Part model, mm, in its own coordinate system. A direction names the side the tool comes from. Round coordinates to 2 decimals unless told otherwise and drop trailing zeros. Write each loop counter-clockwise with the first axis right and the second up, starting at its lowest first coordinate (ties: lowest second). Pieces come first, ordered by that corner, then holes. Notation, with made-up numbers: M 78.25,88.5 L 120.25,88.5 A24 ccw 120.25,101.5 Z; hole C 2,22 d1. An arc over 180 degrees is marked long. Answer as a JSON object with one key per item and string values. Group by question number.
1. Which spindle directions (+Z, -Z, +X, -X, +Y, -Y) get a long thin tool onto all of the face, cutting with end or side? Do faces 4 (the face through (-31.858, -1, 1)), 5 (the face through (9, -21.627, 1)), 6 (the face through (49, 0, 0)). Say none if no direction does.
2. Two-plate mould, pull along X, no slides. Class faces 1 (the face through (-35.154, -0.75, -1.014)), 2 (the face through (47.942, -1, 1)), 3 (the face through (9, 0, -2)): +X half, -X half, draft (parallel to the pull), parting line (faces both ways), or undercut.
3. Band-saw the part on B-B, the plane z = 2. Write the cut outline in (x, y), plus the area to 3 significant figures.
4. Drill centre line: line 1 (X direction, y = -19, z = 1.3). Where is it in solid material? Low to high. Write a range as from..to.
5. Drop flat-ended pins along their axis: pin 1 (1.5 mm diameter, centred on y = -8, z = 1.5, fed in from -X); pin 2 (2.5 mm diameter, centred on x = 51, y = -9, fed in from +Z); pin 3 (3 mm diameter, centred on y = 14, z = 2, fed in from +X). Give the stop position or say it passes through.
6. Band-saw the part on A-A, the plane y = 4. Write the cut outline in (x, z).
from build123d import *

# Parameters (mm, degrees)
SKETCH1_W           = 79.8
SKETCH1_H           = 41.8
BOSS_EXTRUDE1_DEPTH = 3
SKETCH2_W           = 89.8
SKETCH2_H           = 41.8
BOSS_EXTRUDE4_DEPTH = 2
SKETCH3_R           = 1
SKETCH3_R_2         = 0.833875984
CUT_EXTRUDE1_DEPTH  = 2


with BuildPart() as part:
    # Sketch1 → Boss-Extrude1 (new body)
    with BuildSketch(Plane.XY):
        with Locations((8.041732283, -0.726771654)):
            Rectangle(SKETCH1_W, SKETCH1_H)
    extrude(amount=BOSS_EXTRUDE1_DEPTH)

    # Sketch2 → Boss-Extrude4 (add)
    with BuildSketch(Plane(origin=(0, 0, 0), x_dir=(-1, 0, 0), z_dir=(0, 0, -1))):
        with Locations((-8.041732283, -0.726771654)):
            Rectangle(SKETCH2_W, SKETCH2_H)
    extrude(amount=BOSS_EXTRUDE4_DEPTH)

    # Sketch3 → Cut-Extrude1 (cut)
    with BuildSketch(Plane(origin=(0, 0, -2), x_dir=(-1, 0, 0), z_dir=(0, 0, -1))):
        with Locations((-50.441732283, 0)):
            Circle(SKETCH3_R)
        with Locations((34.358267717, -1)):
            Circle(SKETCH3_R_2)
    extrude(amount=-CUT_EXTRUDE1_DEPTH, mode=Mode.SUBTRACT)


solid = part.part
Worked answers:
{
 "1": {"face 4": "+Z, -X, +Y, -Y", "face 5": "+Z, -Z, +X, -X, -Y", "face 6": "+Z, +X, +Y, -Y"},
 "2": {"face 1": "undercut", "face 2": "+X half", "face 3": "draft"},
 "3": {"outline": "M -31.86,-21.63 L 47.94,-21.63 L 47.94,20.17 L -31.86,20.17 Z", "area": "3,340 mm^2"},
 "4": {"line 1": "x = -31.86..47.94"},
 "5": {"pin 1": "stops at x = -31.86", "pin 2": "stops at z = 0", "pin 3": "stops at x = 47.94"},
 "6": {"outline": "M -36.86,-2 L 52.94,-2 L 52.94,0 L 47.94,0 L 47.94,3 L -31.86,3 L -31.86,0 L -36.86,0 Z"}
}
